from build123d import *

# Parameters (mm, degrees)
BOSS_EXTRUDE1_DEPTH = 19.05
SKETCH3_R           = 4
CUT_EXTRUDE1_DEPTH  = 51.899122045
SKETCH4_R           = 4
CUT_EXTRUDE2_DEPTH  = 60.905780189


with BuildPart() as part:
    # Sketch2 → Boss-Extrude1 (new, symmetric)
    with BuildSketch(Plane.XY):
        with BuildLine():
            Line((-15.875, 0), (15.875, 0))
            Line((15.875, 0), (15.875, 50.8))
            Line((15.875, 50.8), (12.7, 50.8))
            ThreePointArc((12.7, 50.8), (10.45493597, 49.87006403), (9.525, 47.625))
            Line((9.525, 47.625), (9.525, 9.525))
            ThreePointArc((9.525, 9.525), (8.59506403, 7.27993597), (6.35, 6.35))
            Line((6.35, 6.35), (-12.7, 6.35))
            ThreePointArc((-12.7, 6.35), (-14.94506403, 5.42006403), (-15.875, 3.175))
            Line((-15.875, 3.175), (-15.875, 0))
        make_face()
    extrude(amount=BOSS_EXTRUDE1_DEPTH, both=True)

    # Sketch3 → Cut-Extrude1 (cut, through all)
    with BuildSketch(Plane(origin=(0, 6.35, 0), x_dir=(1, 0, 0), z_dir=(0, 1, 0))):
        with Locations(Location((-3.175, 9.525, 0), (0, 0, 180))):
            Circle(SKETCH3_R)
        with Locations(Location((-3.175, -9.525, 0), (0, 0, 180))):
            Circle(SKETCH3_R)
    extrude(amount=-CUT_EXTRUDE1_DEPTH, mode=Mode.SUBTRACT)

    # Sketch4 → Cut-Extrude2 (cut, through all)
    with BuildSketch(Plane.ZY.offset(-9.525)):
        with Locations(Location((0, 38.1, 0), (0, 0, 270))):
            Circle(SKETCH4_R)
        with Locations(Location((0, 19.05, 0), (0, 0, 90))):
            Circle(SKETCH4_R)
    extrude(amount=-CUT_EXTRUDE2_DEPTH, mode=Mode.SUBTRACT)


solid = part.part
Verification items for the finished model (mm, model axes). A direction names the side the tool comes from. Coordinates: 2 decimals unless noted, no trailing zeros. Write each loop counter-clockwise with the first axis right and the second up, starting at its lowest first coordinate (ties: lowest second). Pieces come first, ordered by that corner, then holes. Notation, with made-up numbers: (64.5, 3.5) - (121.5, 3.5) arc R9 cw to (121.5, 11.5) - close; hole circle Ø2 at (-28, -3). An arc over 180 degrees is marked (long way). Answer as a JSON object with one key per item and string values.
(1) Cross-section at A-A on y = 19.05. Record the cut outline in (x, z) (3 decimals).
Report:
{"outline": "(9.525, -19.05) - (15.875, -19.05) - (15.875, -4) - (9.525, -4) - close; (9.525, 4) - (15.875, 4) - (15.875, 19.05) - (9.525, 19.05) - close"}
(2) Cross-section at B-B on z = 0. Record the cut outline in (x, y) (3 decimals), plus the area to 3 significant figures.
Report:
{"outline": "(-15.875, 0) - (15.875, 0) - (15.875, 15.05) - (9.525, 15.05) - (9.525, 9.525) arc R3.175 cw to (6.35, 6.35) - (-12.7, 6.35) arc R3.175 ccw to (-15.875, 3.175) - close; (9.525, 23.05) - (15.875, 23.05) - (15.875, 34.1) - (9.525, 34.1) - close; (9.525, 42.1) - (15.875, 42.1) - (15.875, 50.8) - (12.7, 50.8) arc R3.175 ccw to (9.525, 47.625) - close", "area": "380 mm^2"}
(3) Gauge pin test, flat ends, axial feed: pin 1 Ø5 at (y, z) = (38.1, 0) entering from -X; pin 2 Ø2 at (y, z) = (44, -0.5) entering from -X (3 decimals); pin 3 Ø2 at (x, z) = (9.5, -14) entering from +Y; pin 4 Ø10 at (x, z) = (-7.5, 4.5) entering from +Y. Record the tip position at first contact, or that the pin passes through.
Report:
{"pin 1": "through", "pin 2": "x = 9.525", "pin 3": "y = 49.91", "pin 4": "y = 6.35"}
(4) Thickness scan on line 1 along Z through (x, y) = (11, 38.1); line 2 along Y through (x, z) = (14.5, -3); line 3 along Y through (x, z) = (-9.5, -13). Record the ranges inside material, lowest first.
Report:
{"line 1": "-19.05 to -4, 4 to 19.05", "line 2": "0 to 16.4, 21.7 to 35.45, 40.75 to 50.8", "line 3": "0 to 6.35"}
(5) Cross-section at C-C on x = -5. Record the cut outline in (y, z).
Report:
{"outline": "(0, -19.05) - (6.35, -19.05) - (6.35, -13.08) - (0, -13.08) - close; (0, -5.97) - (6.35, -5.97) - (6.35, 5.97) - (0, 5.97) - close; (0, 13.08) - (6.35, 13.08) - (6.35, 19.05) - (0, 19.05) - close"}
(6) Cross-section at D-D on y = 38. Record the cut outline in (x, z) (3 decimals).
Report:
{"outline": "(9.525, -19.05) - (15.875, -19.05) - (15.875, -3.999) - (9.525, -3.999) - close; (9.525, 3.999) - (15.875, 3.999) - (15.875, 19.05) - (9.525, 19.05) - close"}
(7) Tool access check on faces 5 (the flat face through (-15.875, 2, 0)), 6 (the flat face through (-3, 6.35, 0)). Record the directions out of +Z, -Z, +X, -X, +Y, -Y that give a thin tool (end or side, any length) a straight path to the whole face; none if there is none.
Report:
{"face 5": "+Z, -Z, -X, +Y, -Y", "face 6": "+Z, -Z, -X, +Y"}
(8) Mould release check, pull along X, two halves, no side actions. Record for faces 1 (the flat face through (15.875, 25, 0)), 2 (the cylindrical face through (8.62, 7.305, 0.267)), 3 (the cylindrical face through (-2.65, 3.22, 13.49)), 4 (the flat face through (0, 0, 0)): pulls with the +X half, pulls with the -X half, needs draft (parallel to the pull), parting line crosses it, or undercut.
Report:
{"face 1": "pulls with the +X half", "face 2": "pulls with the -X half", "face 3": "undercut", "face 4": "needs draft"}
